from build123d import *

# Parameters (mm, degrees)
F0_W      = 76.2002236371
F0_H      = 83.8200002909
F1_DEPTH  = 19.05
F2_W      = 70.0279923622
F2_H      = 57.9973980784
F3_DEPTH  = 15.24
F4_W      = 13.0012880329
F4_H      = 11.8417413905
F5_DEPTH  = 15.24
F6_W      = 24.8060952872
F6_H      = 10.8370622396
F7_DEPTH  = 15.24
F8_W      = 13.2993943989
F8_H      = 9.0398679234
F9_DEPTH  = 15.24
F10_W     = 64.4978582859
F10_H     = 19.05
F11_DEPTH = 33.02
F12_W     = 64.4978582859
F12_H     = 19.05
F13_DEPTH = 33.02
F14_W     = 142.2402236371
F14_H     = 19.05
F15_DEPTH = 33.02
F16_W     = 135.098611936
F16_H     = 25.4710018635
F17_DEPTH = 15.24
F18_R     = 14.7000934616
F19_DEPTH = 15.24
F20_R     = 11.4164159858
F21_DEPTH = 15.24
F23_DEPTH = 15.24
F24_DEPTH = 25.4


with BuildPart() as f1:
    # F0 (on Top) → F1 (new body)
    with BuildSketch(Plane.XY):
        with Locations((38.1001118185, 22.5878581405)):
            Rectangle(F0_W, F0_H)
    extrude(amount=F1_DEPTH)

    # F2 (on face) → F3 (cut)
    with BuildSketch(Plane(origin=(0, 0, 0), x_dir=(1, 0, 0), z_dir=(0, 0, -1))):
        with Locations((38.089536014, -28.9986990392)):
            Rectangle(F2_W, F2_H)
    extrude(amount=-F3_DEPTH, mode=Mode.SUBTRACT)

    # F4 (on face) → F5 (cut)
    with BuildSketch(Plane(origin=(0, 0, 0), x_dir=(1, 0, 0), z_dir=(0, 0, -1))):
        with Locations((13.4606149513, 9.9389031529)):
            Rectangle(F4_W, F4_H)
    extrude(amount=-F5_DEPTH, mode=Mode.SUBTRACT)

    # F6 (on face) → F7 (cut)
    with BuildSketch(Plane(origin=(0, 0, 0), x_dir=(1, 0, 0), z_dir=(0, 0, -1))):
        with Locations((39.6352009848, 9.4365635775)):
            Rectangle(F6_W, F6_H)
    extrude(amount=-F7_DEPTH, mode=Mode.SUBTRACT)

    # F8 (on face) → F9 (cut)
    with BuildSketch(Plane(origin=(0, 0, 0), x_dir=(1, 0, 0), z_dir=(0, 0, -1))):
        with Locations((66.4538349956, 10.3351607356)):
            Rectangle(F8_W, F8_H)
    extrude(amount=-F9_DEPTH, mode=Mode.SUBTRACT)

    # F10 (on face) → F11 (join)
    with BuildSketch(Plane.YZ.offset(76.2002236371)):
        with Locations((32.248929143, 9.525)):
            Rectangle(F10_W, F10_H)
    extrude(amount=F11_DEPTH)

    # F12 (on face) → F13 (join)
    with BuildSketch(Plane(origin=(0, 0, 0), x_dir=(0, -1, 0), z_dir=(-1, 0, 0))):
        with Locations((-32.248929143, 9.525)):
            Rectangle(F12_W, F12_H)
    extrude(amount=F13_DEPTH)

    # F14 (on face) → F15 (join)
    with BuildSketch(Plane(origin=(0, 64.4978582859, 0), x_dir=(-1, 0, 0), z_dir=(0, 1, 0))):
        with Locations((-38.1001118185, 9.525)):
            Rectangle(F14_W, F14_H)
    extrude(amount=F15_DEPTH)

    # F16 (on face) → F17 (cut)
    with BuildSketch(Plane(origin=(0, 0, 0), x_dir=(1, 0, 0), z_dir=(0, 0, -1))):
        with Locations((37.8726990893, -75.9849250317)):
            Rectangle(F16_W, F16_H)
    extrude(amount=-F17_DEPTH, mode=Mode.SUBTRACT)

    # F18 (on face) → F19 (cut)
    with BuildSketch(Plane(origin=(0, 0, 0), x_dir=(1, 0, 0), z_dir=(0, 0, -1))):
        with Locations((-15.4463164508, -21.2640985847)):
            Circle(F18_R)
    extrude(amount=-F19_DEPTH, mode=Mode.SUBTRACT)

    # F20 (on face) → F21 (cut)
    with BuildSketch(Plane(origin=(0, 0, 0), x_dir=(1, 0, 0), z_dir=(0, 0, -1))):
        with Locations((-14.4130205736, -48.758929143)):
            Circle(F20_R)
    extrude(amount=-F21_DEPTH, mode=Mode.SUBTRACT)

    # F22 (on face) → F23 (cut)
    with BuildSketch(Plane(origin=(0, 0, 0), x_dir=(1, 0, 0), z_dir=(0, 0, -1))):
        Polygon((91.0199095375, -10.8233336359), (82.0573866367, -10.8233336359), (82.0573866367, -54.6272806823), (103.4740805626, -54.6272806823), (103.4740805626, -31.2997968867), (91.0199095375, -31.2997968867), align=None)
    extrude(amount=-F23_DEPTH, mode=Mode.SUBTRACT)

    # F24 (add): a face of the model
    f24_faces = [f1.faces().sort_by_distance(p)[0] for p in [
        (74.3594665405, -9.6610710025, 0),
    ]]
    extrude(f24_faces, amount=F24_DEPTH)


solid = f1.part
Could you check a few things on this model? Use its own coordinates, in mm. A direction names the side the tool comes from. Give positions to 0.01 mm unless a question says otherwise; leave off trailing zeros. Loops run counter-clockwise (first coordinate to the right, second up) from the corner with the lowest first, then second, coordinate; pieces in that order, holes last. Notation, with made-up numbers: M 82,55.25 L 99,55.25 A23 cw 99,85.25 Z; hole C -22.75,55 d4. An arc over 180 degrees is marked long. Answer as a JSON object with one key per item and string values.
Q1. If I drill on probe 1 along Y at (x, z) = (64, 7); probe 2 along Y at (x, z) = (96, -11); probe 3 along Y at (x, z) = (40, -8.5), over which ranges is the centre line in solid material (lowest first)? Write a range as [from, to].
Values found:
{"probe 1": "y = [-19.32, -14.86], [-5.82, 0], [58, 63.25], [88.72, 97.52]", "probe 2": "y = [0, 31.3], [54.63, 63.25], [88.72, 97.52]", "probe 3": "y = [-19.32, -14.86], [-4.02, 0], [58, 63.25], [88.72, 97.52]"}
Q2. Suppose I cut it at A-A, the plane x = 32. List the corners of the cut face in (y, z) for me, plus the area to 3 significant figures.
Values found:
{"outline": "M -19.32,-25.4 L -14.86,-25.4 L -14.86,15.24 L -4.02,15.24 L -4.02,-25.4 L 0,-25.4 L 0,15.24 L 58,15.24 L 58,-25.4 L 63.25,-25.4 L 63.25,15.24 L 88.72,15.24 L 88.72,-25.4 L 97.52,-25.4 L 97.52,19.05 L -19.32,19.05 Z", "area": "1,360 mm²"}
Q3. For P1, Ø15.5, axis at y = -14, z = -13.5, coming from the +X side; P2, Ø8.5, axis at y = -8, z = -2.5, coming from the -X side; P3, Ø2, axis at x = 90, z = -9, coming from the -Y side, each with a flat end and sliding along its axis, tell me the tip position at first contact or that it passes through.
Values found:
{"P1": "stops at x = 76.2", "P2": "stops at x = 0", "P3": "stops at y = 0"}
Q4. Suppose I cut it at C-C, the plane x = 88.5. List the corners of the cut face in (y, z) for me, plus the area to 3 significant figures.
Values found:
{"outline": "M 0,-25.4 L 10.82,-25.4 L 10.82,15.24 L 54.63,15.24 L 54.63,-25.4 L 63.25,-25.4 L 63.25,15.24 L 88.72,15.24 L 88.72,-25.4 L 97.52,-25.4 L 97.52,19.05 L 0,19.05 Z", "area": "1,520 mm²"}
Q5. Suppose I cut it at B-B, the plane y = 66. List the corners of the cut face in (x, z) for me.
Values found:
{"outline": "M -33.02,-25.4 L -29.68,-25.4 L -29.68,15.24 L 105.42,15.24 L 105.42,-25.4 L 109.22,-25.4 L 109.22,19.05 L -33.02,19.05 Z"}
Q6. Suppose I cut it at D-D, the plane z = -14.5. State how many separate pieces and enclosed holes the cut face has, plus the area to 3 significant figures.
Values found:
{"separate pieces": "1", "enclosed holes": "8", "area": "5,530 mm²"}
Q7. For faces 1 (the flat face through (0, -10, -3)), 2 (the flat face through (37, 63.249, -5)), 3 (the flat face through (39, 38, 19.05)), which set-ups out of +Z, -Z, +X, -X, +Y, -Y let a thin tool reach every point of the face, with its end or its side?
Values found:
{"face 1": "+Z, -Z, -X, -Y", "face 2": "-Z", "face 3": "+Z, +X, -X, +Y, -Y"}
Q8. If we mould it in two halves opening along X, with no side actions, what happens to faces 4 (the flat face through (109.22, 48, -3)), 5 (the flat face through (92, 0, -3)), 6 (the flat face through (38, 57.997, -5))? For each: pulls with the +X half, pulls with the -X half, needs draft (parallel to the pull), parting line crosses it, or undercut.
Values found:
{"face 4": "pulls with the +X half", "face 5": "needs draft", "face 6": "undercut"}
